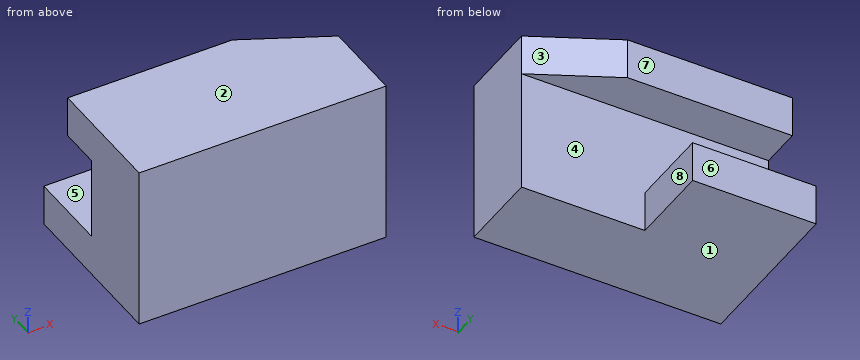
```python
from build123d import *

# Parameters (mm, degrees)
SKETCH_1_W          = 15
SKETCH_1_H          = 5
SKETCH_1_W_2        = 20
SKETCH_1_W_3        = 10
EXTRUDE_1_DEPTH     = 10
SKETCH_1_3_W        = 20
SKETCH_1_3_H        = 5
SKETCH_1_3_W_2      = 10
EXTRUDE_2_DEPTH     = 15
SKETCH_1_4_W        = 15
SKETCH_1_4_H        = 5
EXTRUDE_3_DEPTH     = 20
CUT_EXTRUDE_1_DEPTH = 20


with BuildPart() as part:
    # Sketch 1 → Extrude 1 (new body)
    with BuildSketch(Plane(origin=(0, 0, 0), x_dir=(1, 0, 0), z_dir=(0, 1, 0))):
        with Locations((-7.5, 7.5)):
            Rectangle(SKETCH_1_W, SKETCH_1_H)
        Polygon((15, -5), (15, 10), (0, 10), (0, 5), (-15, 5), (-15, -5), (5, -5), align=None)
        with Locations((-5, -7.5)):
            Rectangle(SKETCH_1_W_2, SKETCH_1_H)
        with Locations((10, -7.5)):
            Rectangle(SKETCH_1_W_3, SKETCH_1_H)
    extrude(amount=EXTRUDE_1_DEPTH)

    # Sketch 1_3 → Extrude 2 (add)
    with BuildSketch(Plane(origin=(0, 0, 0), x_dir=(1, 0, 0), z_dir=(0, 1, 0))):
        with Locations((-5, -7.5)):
            Rectangle(SKETCH_1_3_W, SKETCH_1_3_H)
        with Locations((10, -7.5)):
            Rectangle(SKETCH_1_3_W_2, SKETCH_1_3_H)
    extrude(amount=EXTRUDE_2_DEPTH)

    # Sketch 1_4 → Extrude 3 (add)
    with BuildSketch(Plane(origin=(0, 0, 0), x_dir=(1, 0, 0), z_dir=(0, 1, 0))):
        with Locations((-7.5, 7.5)):
            Rectangle(SKETCH_1_4_W, SKETCH_1_4_H)
    extrude(amount=EXTRUDE_3_DEPTH)

    # Sketch 2 → Cut-Extrude 1 (cut)
    with BuildSketch(Plane.XY.offset(10)):
        Polygon((5, 15), (15, 10), (15, 15), align=None)
    extrude(amount=-CUT_EXTRUDE_1_DEPTH, mode=Mode.SUBTRACT)


solid = part.part
```
Can you work these out from the model? Positions are in its coordinate system, mm. Face numbers are marked on the shaded views. A direction names the side the tool comes from. Give positions to 0.01 mm unless a question says otherwise; leave off trailing zeros. Loops run counter-clockwise (first coordinate to the right, second up) from the corner with the lowest first, then second, coordinate; pieces in that order, holes last. Notation, with made-up numbers: M -32.75,38 L 1.25,38 A25 ccw 1.25,72 Z; hole C 50.5,46.25 d5. An arc over 180 degrees is marked long. One line per item, written item: value.
(1) Will these pins go through, and if not, where does the flat tip stop? pin 1 (1.5 mm diameter, centred on x = -3, z = 6.5, fed in from +Y); pin 2 (1.5 mm diameter, centred on y = 15, z = -7.5, fed in from +X); pin 3 (1.5 mm diameter, centred on y = 16, z = 6.5, fed in from -X).
Returned:
pin 1: y = 15
pin 2: x = 0
pin 3: through
(2) Suppose I cut it at A-A on y = 12. List the corners of the cut face in (x, z) for me, plus the area to 3 significant figures.
Returned:
outline: M -15,-10 L 0,-10 L 0,-5 L -15,-5 Z; M -15,5 L 11,5 L 11,10 L -15,10 Z
area: 205 mm^2
(3) Which directions (+Z, -Z, +X, -X, +Y, -Y) give clear straight access to the entire face, cutting with the end or side of a thin tool? Please do the marked faces 5, 6, 7 and 8.
Returned:
face 5: +X, -X, +Y
face 6: +Z, -Z, +X, -X, +Y
face 7: +Z, +X, -X, +Y
face 8: -Z, +X, +Y
(4) Suppose I cut it at C-C on z = 5.5. List the corners of the cut face in (x, y) for me, plus the area to 3 significant figures.
Returned:
outline: M -15,0 L 15,0 L 15,10 L 5,15 L -15,15 Z
area: 425 mm^2
(5) I need wall thicknesses on line 1 (Y direction, x = 10.5, z = -6); line 2 (Y direction, x = 0.25, z = 5.5); line 3 (Z direction, x = 2.75, y = 10.5). Which ranges of each line are inside material? Lowest first, please.
Returned:
line 1: 0 to 10
line 2: 0 to 15
line 3: 5 to 10
(6) Suppose I cut it at B-B on x = -8. List the corners of the cut face in (y, z) for me.
Returned:
outline: M 0,-10 L 20,-10 L 20,-5 L 10,-5 L 10,5 L 15,5 L 15,10 L 0,10 Z
(7) Suppose I cut it at D-D on y = 16.25. List the corners of the cut face in (x, z) for me, plus the area to 3 significant figures.
Returned:
outline: M -15,-10 L 0,-10 L 0,-5 L -15,-5 Z
area: 75.0 mm^2
(8) We'd pull the mould along Z, two halves only. Please class the marked faces 1, 2, 3 and 4: released by +Z, released by -Z, zero draft, split by the parting line, or undercut.
Returned:
face 1: released by -Z
face 2: released by +Z
face 3: zero draft
face 4: undercut
